from build123d import *

# Parameters (mm, degrees)
SKETCH1_W           = 150
SKETCH1_H           = 500
BOSS_EXTRUDE1_DEPTH = 30
SKETCH2_W           = 100
SKETCH2_H           = 50
BOSS_EXTRUDE2_DEPTH = 150
SKETCH3_W           = 100
SKETCH3_H           = 50
BOSS_EXTRUDE3_DEPTH = 150
FILLET1_R           = 5
SKETCH4_R           = 14.383133374
SKETCH4_R_2         = 14.814559663
CUT_EXTRUDE1_DEPTH  = 538.959106253


with BuildPart() as part:
    # Sketch1 → Boss-Extrude1 (new body)
    with BuildSketch(Plane.XY):
        with Locations((75, 250)):
            Rectangle(SKETCH1_W, SKETCH1_H)
    extrude(amount=BOSS_EXTRUDE1_DEPTH)

    # Sketch2 → Boss-Extrude2 (add)
    with BuildSketch(Plane.ZY):
        with Locations((80, 475)):
            Rectangle(SKETCH2_W, SKETCH2_H)
    extrude(amount=-BOSS_EXTRUDE2_DEPTH)

    # Sketch3 → Boss-Extrude3 (add)
    with BuildSketch(Plane.ZY):
        with Locations((80, 25)):
            Rectangle(SKETCH3_W, SKETCH3_H)
    extrude(amount=-BOSS_EXTRUDE3_DEPTH)

    # Fillet1
    fillet1_edges = [part.edges().sort_by_distance(p)[0] for p in [
        (75, 500, 0),
        (75, 0, 0),
    ]]
    fillet(fillet1_edges, radius=FILLET1_R)

    # Sketch4 → Cut-Extrude1 (cut, through all)
    with BuildSketch(Plane(origin=(0, 500, 0), x_dir=(1, 0, 0), z_dir=(0, 1, 0))):
        with Locations(Location((37.5, -92.5, 0), (0, 0, 270))):
            Circle(SKETCH4_R)
        with Locations(Location((112.5, -92.5, 0), (0, 0, 270))):
            Circle(SKETCH4_R_2)
    extrude(amount=-CUT_EXTRUDE1_DEPTH, mode=Mode.SUBTRACT)


solid = part.part
The model under review builds one solid part; all positions refer to its coordinate system, in mm. A direction names the side the tool comes from. Round coordinates to 2 decimals unless told otherwise and drop trailing zeros. Loops run counter-clockwise (first coordinate to the right, second up) from the corner with the lowest first, then second, coordinate; pieces in that order, holes last. Notation, with made-up numbers: (45.5, -0.75) -> (81.5, -0.75) arc R23 cw to (81.5, 18.25) -> close; hole circle Ø2 at (-24, -35). An arc over 180 degrees is marked (long way). Return JSON: item names as keys, results as strings.
(1) Add section C-C on z = 92.5. Write out the cut boundary in (x, y).
Solved:
{"outline": "(0, 0) -> (23.12, 0) -> (23.12, 50) -> (0, 50) -> close; (0, 450) -> (23.12, 450) -> (23.12, 500) -> (0, 500) -> close; (51.88, 0) -> (97.69, 0) -> (97.69, 50) -> (51.88, 50) -> close; (51.88, 450) -> (97.69, 450) -> (97.69, 500) -> (51.88, 500) -> close; (127.31, 0) -> (150, 0) -> (150, 50) -> (127.31, 50) -> close; (127.31, 450) -> (150, 450) -> (150, 500) -> (127.31, 500) -> close"}
(2) For faces 1 (the flat face through (74, 50, 79)), 2 (the flat face through (0, 254, 21)), list the 3-axis set-ups (+Z, -Z, +X, -X, +Y, -Y) from which the entire face can be reached by the end or side of a thin tool; tool diameter is ignored.
Solved:
{"face 1": "+Z, +X, -X", "face 2": "+Z, -Z, -X, +Y, -Y"}
(3) Add section A-A on z = 57. Write out the cut boundary in (x, y).
Solved:
{"outline": "(0, 0) -> (150, 0) -> (150, 50) -> (0, 50) -> close; (0, 450) -> (150, 450) -> (150, 500) -> (0, 500) -> close"}
(4) For line 1 (X direction, y = 481, z = 92.5); line 2 (Y direction, x = 28, z = 124); line 3 (Z direction, x = 112, y = 28), list the stretches that pass through material, from the lowest coordinate up.
Solved:
{"line 1": "0 to 23.12, 51.88 to 97.69, 127.31 to 150", "line 2": "0 to 50, 450 to 500", "line 3": "0 to 77.69, 107.31 to 130"}
(5) Add section B-B on x = 37.5. Write out the cut boundary in (y, z).
Solved:
{"outline": "(0, 5) arc R5 ccw to (5, 0) -> (495, 0) arc R5 ccw to (500, 5) -> (500, 78.12) -> (450, 78.12) -> (450, 30) -> (50, 30) -> (50, 78.12) -> (0, 78.12) -> close; (0, 106.88) -> (50, 106.88) -> (50, 130) -> (0, 130) -> close; (450, 106.88) -> (500, 106.88) -> (500, 130) -> (450, 130) -> close"}
(6) For pin 1 (18 mm diameter, centred on x = 112.5, z = 92.5, fed in from -Y), flat-tipped, find the tip position at first contact; note if it passes through.
Solved:
{"pin 1": "through"}
(7) The part is to be moulded in two halves that separate along X. For faces 3 (the cylindrical face through (106.826, 25.35, 106.185)), 4 (the flat face through (74, 0, 67)), 5 (the flat face through (150, 254, 21)), say which applies: released by +X, released by -X, zero draft, split by the parting line, or undercut.
Solved:
{"face 3": "undercut", "face 4": "zero draft", "face 5": "released by +X"}
(8) Add section D-D on y = 58. Write out the cut boundary in (x, z), plus the area to 3 significant figures.
Solved:
{"outline": "(0, 0) -> (150, 0) -> (150, 30) -> (0, 30) -> close", "area": "4,500 mm2"}
